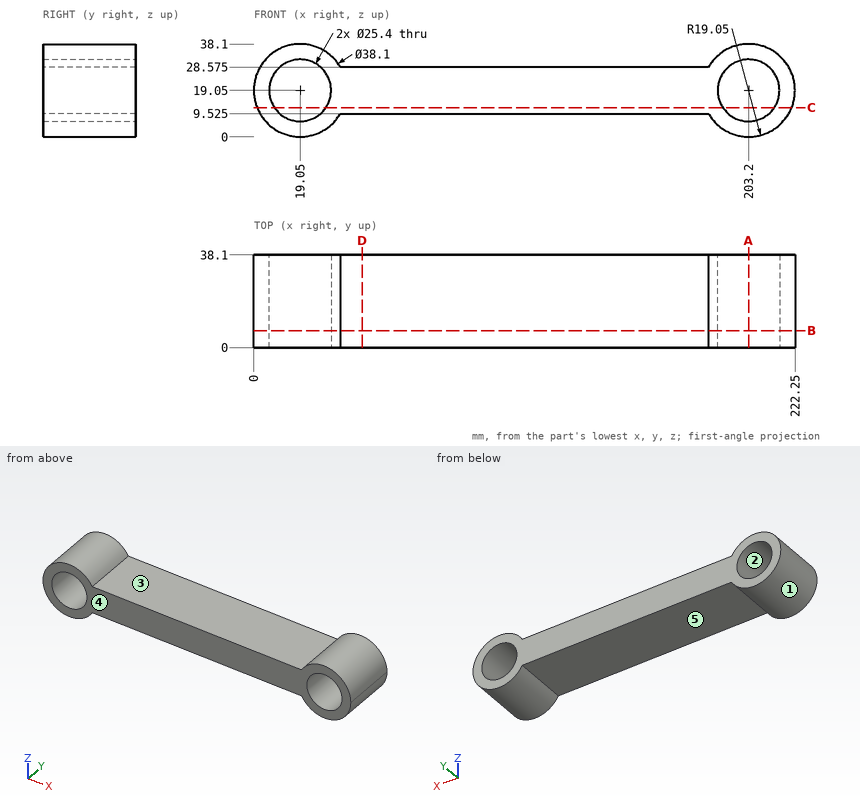
Study the drawing (mm; zero at the part's minimum x, y, z) and answer. A direction names the side the tool comes from. Give positions to 0.01 mm unless a question says otherwise; leave off trailing zeros. Loops run counter-clockwise (first coordinate to the right, second up) from the corner with the lowest first, then second, coordinate; pieces in that order, holes last. Notation, with made-up numbers: (-1.5, -39) - (14.5, -39) arc R16 ccw to (14.5, -18) - close; hole circle Ø3 at (-34.5, -30.5). An arc over 180 degrees is marked (long way). Answer in a Markdown table with one row per item. Add a question column.
Q1. The part is cut by section C-C (z = 12). Determine the outline of the cut face in (x, y), and give its area (3 significant figures).
Q2. The part is cut by section D-D (x = 44.5). Determine the outline of the cut face in (y, z) (3 decimals), and give its area (3 significant figures).
Q3. A tool of negligible diameter and unlimited length cuts with its end or side. For the marked faces 4 and 5, from which of +Z, -Z, +X, -X, +Y, -Y can it reach the whole face along a straight path? Write none if from no direction.
Q4. Each of these flat-tipped pins is pushed along its axis until it touches: P1, Ø6, axis at x = 119, y = 16.5, coming from the +Z side (3 decimals); P2, Ø3, axis at x = 185.5, y = 17.5, coming from the -Z side; P3, Ø8, axis at y = 24.5, z = 13, coming from the +X side. Where does it stop, or does it pass through?
Q5. Determine the mould class of the marked faces 1, 2 and 3 for opening direction Z: released by +Z, released by -Z, zero draft, split by the parting line, or undercut.
Q6. Consider line 1 along X through (y, z) = (4.5, 20); line 2 along X through (y, z) = (17.5, 23.5); line 3 along X through (y, z) = (35.5, 30.5). Determine where each line is inside the solid, lowest interval first.
Q7. The part is cut by section A-A (x = 203.2). Determine the outline of the cut face in (y, z), and give its area (3 significant figures).
Q8. The part is cut by section B-B (y = 7). Determine the outline of the cut face in (x, z) (3 decimals).
Solution:
| question | item | result |
|---|---|---|
| 1 | outline | (1.35, 0) - (8.49, 0) - (8.49, 38.1) - (1.35, 38.1) - close; (29.61, 0) - (192.64, 0) - (192.64, 38.1) - (29.61, 38.1) - close; (213.76, 0) - (220.9, 0) - (220.9, 38.1) - (213.76, 38.1) - close |
| 1 | area | 6,750 mm² |
| 2 | outline | (0, 9.525) - (38.1, 9.525) - (38.1, 28.575) - (0, 28.575) - close |
| 2 | area | 726 mm² |
| 3 | face 4 | +Z, -Z, +X, -X, -Y |
| 3 | face 5 | -Z, +Y, -Y |
| 4 | P1 | stops at z = 28.575 |
| 4 | P2 | stops at z = 9.03 |
| 4 | P3 | stops at x = 222.14 |
| 5 | face 1 | split by the parting line |
| 5 | face 2 | undercut |
| 5 | face 3 | released by +Z |
| 6 | line 1 | x = 0.02 to 6.39, 31.71 to 190.54, 215.86 to 222.23 |
| 6 | line 2 | x = 0.53 to 7.16, 30.94 to 191.31, 215.09 to 221.72 |
| 6 | line 3 | x = 3.83 to 13.56, 24.54 to 34.27, 187.98 to 197.71, 208.69 to 218.42 |
| 7 | outline | (0, 0) - (38.1, 0) - (38.1, 6.35) - (0, 6.35) - close; (0, 31.75) - (38.1, 31.75) - (38.1, 38.1) - (0, 38.1) - close |
| 7 | area | 484 mm² |
| 8 | outline | (35.548, 9.525) - (186.702, 9.525) arc R19.05 ccw (long way) to (186.702, 28.575) - (35.548, 28.575) arc R19.05 ccw (long way) to start; hole circle Ø25.4 at (19.05, 19.05); hole circle Ø25.4 at (203.2, 19.05) |
